Input: dimensioned drawing with shaded views. Units: mm. Origin: part minimum x, y, z. Coordinates: 2 decimals unless noted, no trailing zeros. Write each loop counter-clockwise with the first axis right and the second up, starting at its lowest first coordinate (ties: lowest second). Pieces come first, ordered by that corner, then holes. Notation, with made-up numbers: M -23.5,-11.75 L 30.5,-11.75 A28 cw 30.5,11.25 Z; hole C 15.5,70 d6. An arc over 180 degrees is marked long. Write each question's results on one line, items separated by ' | '. Start each with the question number.
1. Section query A-A, the plane x = 17.5. Output: boundary loops of the cut face in (y, z) (1 decimal).
2. Ray query, probe 1 along X at (y, z) = (12.5, 13) (1 decimal); probe 2 along X at (y, z) = (4.5, 13.75); probe 3 along Y at (x, z) = (17, 2.25). Return the intervals inside material, ascending.
3. Pull-direction query (X, two-part tool) for the marked faces 1, 2 and 3; classes: +X half, -X half, draft (parallel to the pull), parting line (faces both ways), or undercut.
4. First-contact query: pin 1 (8 mm diameter, centred on x = 15.07, z = 12.92, fed in from +Y); pin 2 (8 mm diameter, centred on y = 2.5, z = 5.5, fed in from -X). Flat tips, straight axial feed; report the tip coordinate or a pass-through.
5. Section query B-B, the plane z = 10.25. Output: boundary loops of the cut face in (x, y) (1 decimal), and give its area (3 significant figures).
6. Section query C-C, the plane x = 9. Output: boundary loops of the cut face in (y, z), and give its area (3 significant figures).
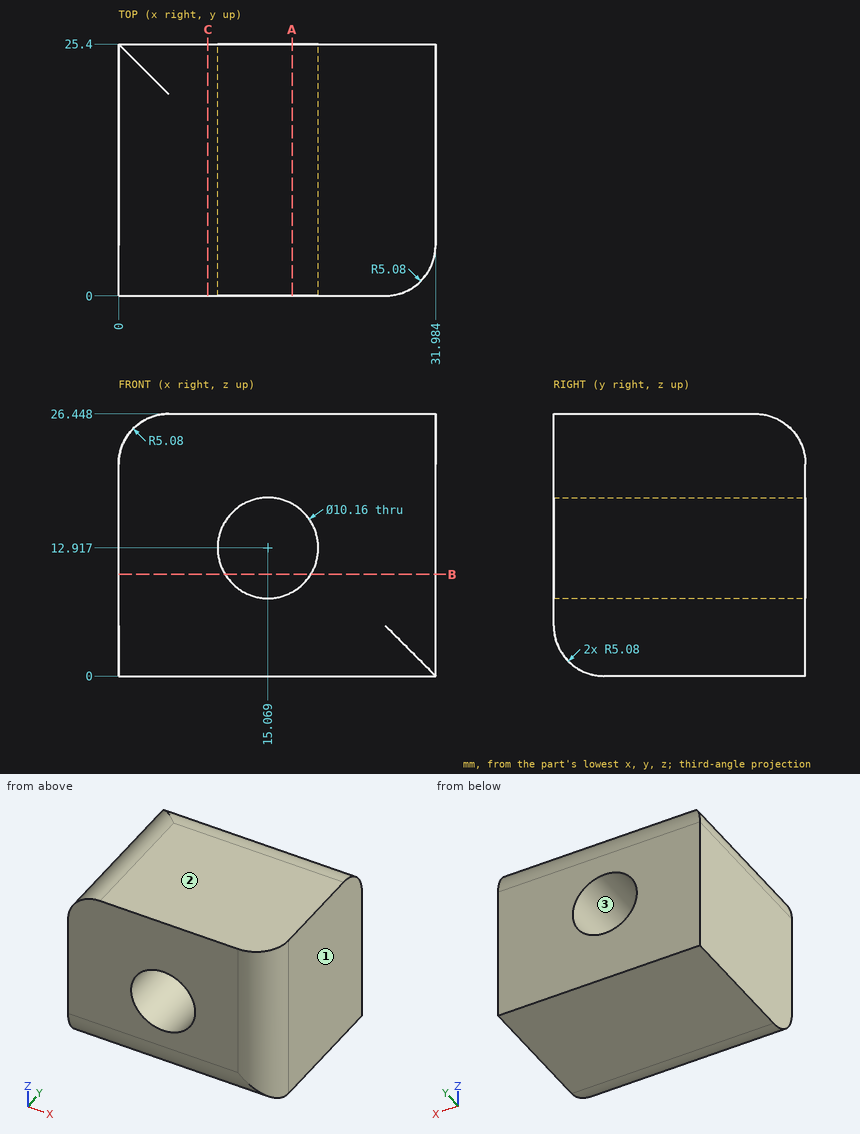
Answer:
1) outline: M 0,5.1 A5.1 ccw 5.1,0 L 25.4,0 L 25.4,8.5 L 0,8.5 Z; M 0,17.4 L 25.4,17.4 L 25.4,21.4 A5.1 ccw 20.3,26.4 L 0,26.4 Z
2) probe 1: 0 to 10, 20.1 to 32 | probe 2: 0 to 10.06, 20.08 to 31.95 | probe 3: 0.86 to 25.4
3) face 1: +X half | face 2: draft | face 3: undercut
4) pin 1: through | pin 2: x = 0
5) outline: M 0,0 L 10.7,0 L 10.7,25.4 L 0,25.4 Z; M 19.4,0 L 26.9,0 A5.1 ccw 32,5.1 L 32,25.4 L 19.4,25.4 Z | area: 587 mm^2
6) outline: M 0,5.08 A5.08 ccw 5.08,0 L 25.4,0 L 25.4,21.37 A5.08 ccw 20.32,26.45 L 0,26.45 Z | area: 661 mm^2
